Geometry: see drawing. Coordinates: mm, zero at the bounding-box minimum. A direction names the side the tool comes from. Round coordinates to 2 decimals unless told otherwise and drop trailing zeros. Loops run counter-clockwise (first coordinate to the right, second up) from the corner with the lowest first, then second, coordinate; pieces in that order, holes last. Notation, with made-up numbers: M -17,-5 L -2,-5 A24 ccw -2,6 Z; hole C 36,73.25 d8. An arc over 180 degrees is marked long. Answer as a JSON object with one key per item and string values.
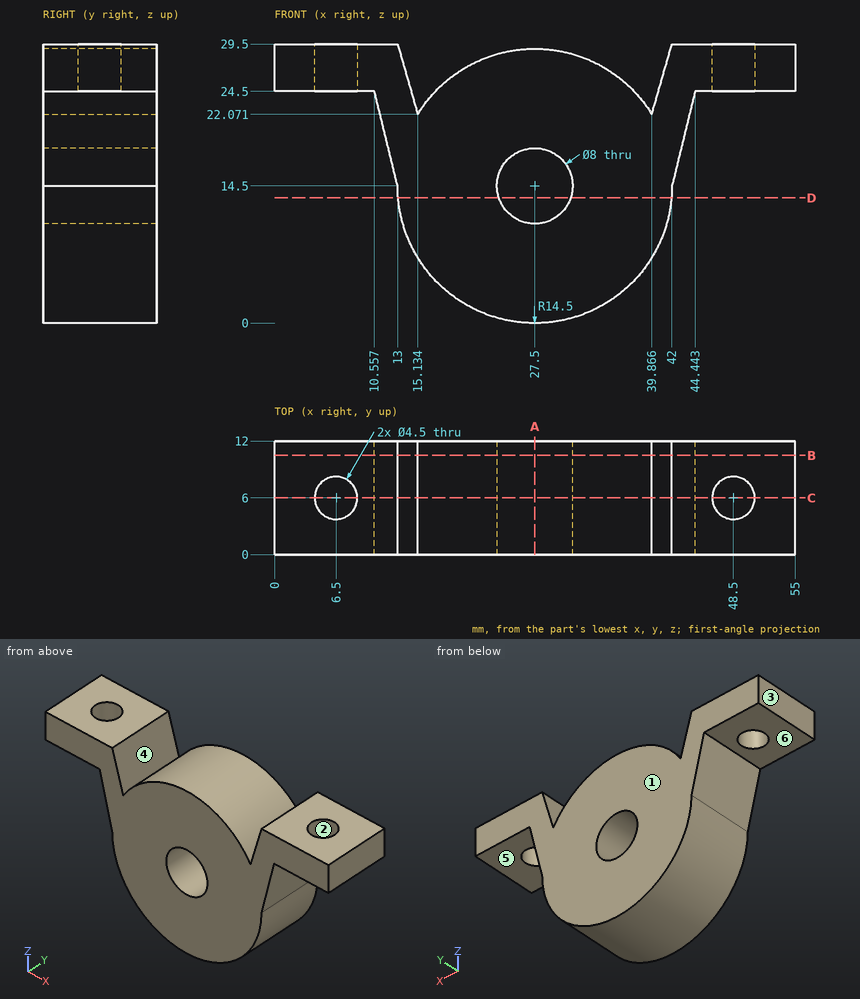
1) Ray query, line 1 (X direction, y = 6.75, z = 14.25); line 2 (Y direction, x = 6.5, z = 26.1); line 3 (Z direction, x = 27.5, y = 9). Return the intervals inside material, ascending.
Results:
{"line 1": "13 to 23.51, 31.49 to 42", "line 2": "0 to 3.75, 8.25 to 12", "line 3": "0 to 10.5, 18.5 to 29"}
2) Section query D-D (z = 13.25). Return the cut outline in (x, y).
Results:
{"outline": "M 13.05,0 L 23.7,0 L 23.7,12 L 13.05,12 Z; M 31.3,0 L 41.95,0 L 41.95,12 L 31.3,12 Z"}
3) Reachability of the marked faces 4, 5 and 6 from +Z, -Z, +X, -X, +Y, -Y: full face, straight path, thin tool, end or side. Return the list, or none.
Results:
{"face 4": "+Z, +Y, -Y", "face 5": "-Z, +X, +Y, -Y", "face 6": "-Z, -X, +Y, -Y"}
4) Section query C-C (y = 6). Return the cut outline in (x, z), and give its area (3 significant figures).
Results:
{"outline": "M 0,24.5 L 4.25,24.5 L 4.25,29.5 L 0,29.5 Z; M 8.75,24.5 L 10.56,24.5 L 13,14.5 A14.5 ccw 42,14.5 L 44.44,24.5 L 46.25,24.5 L 46.25,29.5 L 42,29.5 L 39.87,22.07 A14.5 ccw 15.13,22.07 L 13,29.5 L 8.75,29.5 Z; M 50.75,24.5 L 55,24.5 L 55,29.5 L 50.75,29.5 Z; hole C 27.5,14.5 d8", "area": "746 mm2"}
5) Pin query (flat end, axial travel): P1, Ø5, axis at y = 6.5, z = 18, coming from the +X side (1 decimal); P2, Ø3, axis at x = 5.5, y = 4, coming from the -Z side; P3, Ø2, axis at x = 18.5, y = 9, coming from the +Z side. Return the tip coordinate at first contact, or that it passes through.
Results:
{"P1": "x = 43.5", "P2": "z = 24.5", "P3": "z = 26.59"}
6) Pull-direction query (Y, two-part tool) for the marked faces 1, 2 and 3; classes: +Y half, -Y half, draft (parallel to the pull), parting line (faces both ways), or undercut.
Results:
{"face 1": "+Y half", "face 2": "undercut", "face 3": "draft"}
7) Section query B-B (y = 10.5). Return the cut outline in (x, z).
Results:
{"outline": "M 0,24.5 L 10.56,24.5 L 13,14.5 A14.5 ccw 42,14.5 L 44.44,24.5 L 55,24.5 L 55,29.5 L 42,29.5 L 39.87,22.07 A14.5 ccw 15.13,22.07 L 13,29.5 L 0,29.5 Z; hole C 27.5,14.5 d8"}
8) Section query A-A (x = 27.5). Return the cut outline in (y, z).
Results:
{"outline": "M 0,0 L 12,0 L 12,10.5 L 0,10.5 Z; M 0,18.5 L 12,18.5 L 12,29 L 0,29 Z"}
